Verification items for the finished model (mm, model axes). A direction names the side the tool comes from. Give positions to 0.01 mm unless a question says otherwise; leave off trailing zeros. Loops run counter-clockwise (first coordinate to the right, second up) from the corner with the lowest first, then second, coordinate; pieces in that order, holes last. Notation, with made-up numbers: (-2, 13.5) -> (28, 13.5) arc R30 cw to (28, 35.5) -> close; hole circle Ø4 at (54, 28). An arc over 180 degrees is marked (long way). Use one line per item in the form item = value. Start each with the question number.
from build123d import *

# Parameters (mm, degrees)
SKETCH_1_W          = 28.9
SKETCH_1_H          = 20
SKETCH_1_R          = 1.5
EXTRUDE_1_DEPTH     = 2
EXTRUDE_2_DEPTH     = 20
SKETCH_4_R          = 6
CUT_EXTRUDE_1_DEPTH = 10


with BuildPart() as part:
    # 草图1 → 凸台-拉伸1 (new body)
    with BuildSketch(Plane.XY):
        with Locations((18.138262449, 35.158029485)):
            Rectangle(SKETCH_1_W, SKETCH_1_H)
        with Locations((27.588262449, 42.658029485)):
            Circle(SKETCH_1_R, mode=Mode.SUBTRACT)
        with Locations((8.688262449, 42.658029485)):
            Circle(SKETCH_1_R, mode=Mode.SUBTRACT)
        with Locations((8.688262449, 27.658029485)):
            Circle(SKETCH_1_R, mode=Mode.SUBTRACT)
        with Locations((27.588262449, 27.658029485)):
            Circle(SKETCH_1_R, mode=Mode.SUBTRACT)
    extrude(amount=EXTRUDE_1_DEPTH)

    # 草图2 → 凸台-拉伸2 (add)
    with BuildSketch(Plane.XY.offset(2)):
        Polygon((3.688262449, 35.158029485), (3.688262449, 37.158029485), (32.588262449, 37.158029485), (32.588262449, 33.158029485), (3.688262449, 33.158029485), align=None)
    extrude(amount=EXTRUDE_2_DEPTH)

    # 草图4 → 切除-拉伸1 (cut)
    with BuildSketch(Plane.XZ.offset(-33.158029485)):
        with Locations((18.138262449, 12)):
            Circle(SKETCH_4_R)
    extrude(amount=-CUT_EXTRUDE_1_DEPTH, mode=Mode.SUBTRACT)


solid = part.part
Item 1: Sectioned sample at B-B, the plane x = 16.25. Enter the section's corners in (y, z), and give its area (3 significant figures).
Item 2: Sectioned sample at C-C, the plane y = 36.75. Enter the section's corners in (x, z).
Item 3: Gauge pin test, flat ends, axial feed: pin 1 Ø1 at (x, y) = (13, 29.5) entering from +Z; pin 2 Ø6 at (x, z) = (25, 14) entering from +Y; pin 3 Ø1.5 at (x, z) = (8.5, 10) entering from -Y. Record the tip position at first contact, or that the pin passes through.
Item 4: Sectioned sample at D-D, the plane x = 13. Enter the section's corners in (y, z), and give its area (3 significant figures).
Item 5: Draft check along Y on faces 1 (the cylindrical face through (26.48, 28.67, 0.99)), 2 (the flat face through (18, 25.158, 1)), 3 (the flat face through (18, 35, 22)). Enter one of: +Y half, -Y half, draft (parallel to the pull), parting line (faces both ways), or undercut.
Item 6: Material ranges on line 1 (Z direction, x = 5.25, y = 26.5); line 2 (Y direction, x = 28, z = 14); line 3 (Z direction, x = 14.25, y = 36.5), recorded low to high.
Item 7: Sectioned sample at A-A, the plane z = 12. Enter the section's corners in (x, y), and give its area (3 significant figures).
Item 8: Tool access check on faces 4 (the flat face through (18, 29, 2)), 5 (the cylindrical face through (27.263, 41.194, 0.986)), 6 (the flat face through (18, 41, 2)). Record the directions out of +Z, -Z, +X, -X, +Y, -Y that give a thin tool (end or side, any length) a straight path to the whole face; none if there is none.
Outcome:
q1.outline = (25.16, 0) -> (45.16, 0) -> (45.16, 2) -> (37.16, 2) -> (37.16, 6.3) -> (33.16, 6.3) -> (33.16, 2) -> (25.16, 2) -> close; (33.16, 17.7) -> (37.16, 17.7) -> (37.16, 22) -> (33.16, 22) -> close
q1.area = 74.4 mm^2
q2.outline = (3.69, 0) -> (32.59, 0) -> (32.59, 22) -> (3.69, 22) -> close; hole circle Ø12 at (18.14, 12)
q3.pin_1 = 2
q3.pin_2 = 37.16
q3.pin_3 = 33.16
q4.outline = (25.16, 0) -> (45.16, 0) -> (45.16, 2) -> (37.16, 2) -> (37.16, 8.9) -> (33.16, 8.9) -> (33.16, 2) -> (25.16, 2) -> close; (33.16, 15.1) -> (37.16, 15.1) -> (37.16, 22) -> (33.16, 22) -> close
q4.area = 95.2 mm^2
q5.face_1 = undercut
q5.face_2 = -Y half
q5.face_3 = draft
q6.line_1 = 0 to 2
q6.line_2 = 33.16 to 37.16
q6.line_3 = 0 to 7.43, 16.57 to 22
q7.outline = (3.69, 33.16) -> (12.14, 33.16) -> (12.14, 37.16) -> (3.69, 37.16) -> close; (24.14, 33.16) -> (32.59, 33.16) -> (32.59, 37.16) -> (24.14, 37.16) -> close
q7.area = 67.6 mm^2
q8.face_4 = +Z, +X, -X, -Y
q8.face_5 = +Z, -Z
q8.face_6 = +Z, +X, -X, +Y
